Design review of the part shown in the three views and the two pictorial views. Dimensions are in mm from the part's minimum x, y and z. A direction names the side the tool comes from. Round coordinates to 2 decimals unless told otherwise and drop trailing zeros. Order: outer loops, then holes, each group sorted by start corner. A loop starts at its lowest first (then second) coordinate and runs counter-clockwise, first axis right, second up.
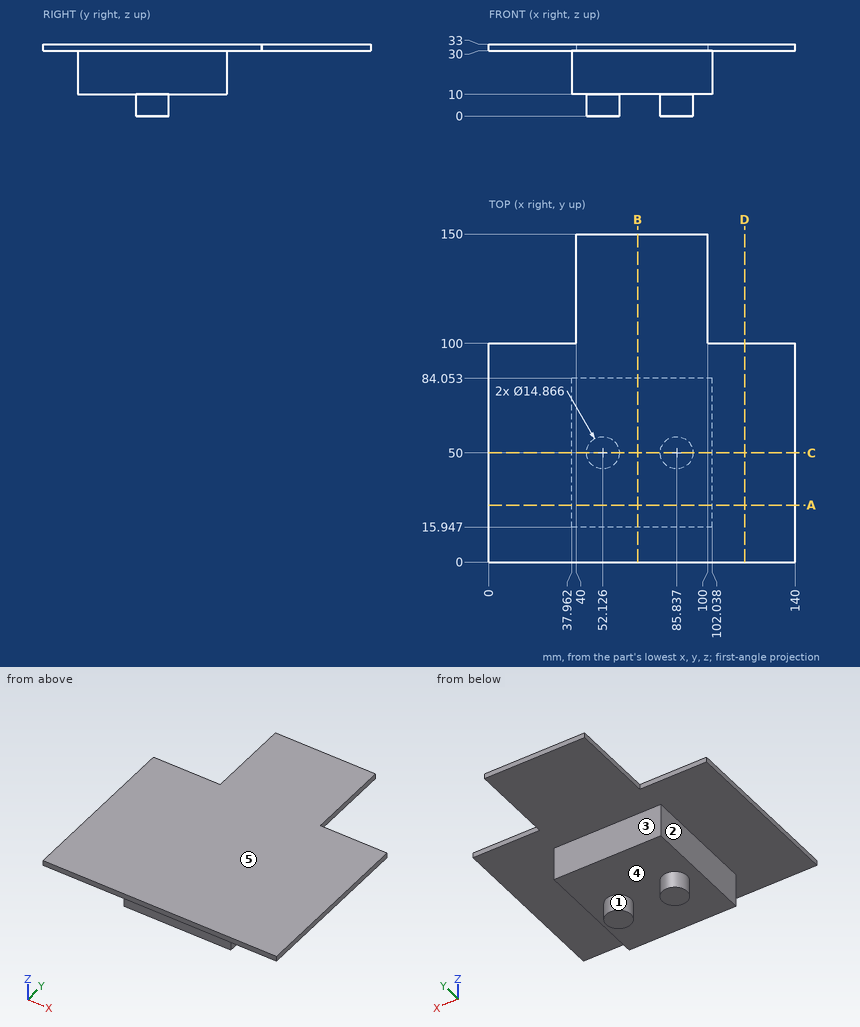
(1) Consider section C-C (y = 50). Write out the cut boundary in (x, z) (1 decimal), and give its area (3 significant figures).
Data:
outline: (0, 30) - (38, 30) - (38, 10) - (44.7, 10) - (44.7, 0) - (59.6, 0) - (59.6, 10) - (78.4, 10) - (78.4, 0) - (93.3, 0) - (93.3, 10) - (102, 10) - (102, 30) - (140, 30) - (140, 33) - (0, 33) - close
area: 2,000 mm2
(2) To check wall thickness, follow probe 1 along Y at (x, z) = (92.5, 24); probe 2 along Z at (x, y) = (30, 56); probe 3 along Z at (x, y) = (68, 70). State the ranges of each line that lie inside material, in increasing order.
Data:
probe 1: y = 15.95 to 84.05
probe 2: z = 30 to 33
probe 3: z = 10 to 33
(3) Consider section A-A (y = 26). Write out the cut boundary in (x, z), and give its area (3 significant figures).
Data:
outline: (0, 30) - (37.96, 30) - (37.96, 10) - (102.04, 10) - (102.04, 30) - (140, 30) - (140, 33) - (0, 33) - close
area: 1,700 mm2
(4) Draft analysis for pull direction X (two halves, no side actions). For the marked faces 1, 2 and 3, state which applies: pulls with the +X half, pulls with the -X half, needs draft (parallel to the pull), parting line crosses it, or undercut.
Data:
face 1: undercut
face 2: pulls with the -X half
face 3: needs draft
(5) Consider section B-B (x = 68). Write out the cut boundary in (y, z), and give its area (3 significant figures).
Data:
outline: (0, 30) - (15.95, 30) - (15.95, 10) - (84.05, 10) - (84.05, 30) - (150, 30) - (150, 33) - (0, 33) - close
area: 1,810 mm2
(6) Insertion check: pin 1 (1.5 mm diameter, centred on y = 116, z = 31, fed in from -X); pin 2 (16 mm diameter, centred on y = 34.5, z = 16, fed in from +X); pin 3 (1.5 mm diameter, centred on x = 16.5, z = 31.5, fed in from +Y). Each pin has a flat end and moves straight along its axis. Give the tip position at first contact, or say it passes through.
Data:
pin 1: stops at x = 40
pin 2: stops at x = 102.04
pin 3: stops at y = 100
(7) Consider section D-D (x = 117). Write out the cut boundary in (y, z).
Data:
outline: (0, 30) - (100, 30) - (100, 33) - (0, 33) - close
(8) For the marked faces 4 and 5, list the 3-axis set-ups (+Z, -Z, +X, -X, +Y, -Y) from which the entire face can be reached by the end or side of a thin tool; tool diameter is ignored.
Data:
face 4: -Z
face 5: +Z, +X, -X, +Y, -Y
